Verification items for the finished model (mm, model axes). A direction names the side the tool comes from. Coordinates: 2 decimals unless noted, no trailing zeros. Order: outer loops, then holes, each group sorted by start corner. A loop starts at its lowest first (then second) coordinate and runs counter-clockwise, first axis right, second up. Notation, with made-up numbers: M 57,-6.5 L 65,-6.5 A12 ccw 65,-2.5 Z; hole C -34.75,56 d1. An arc over 180 degrees is marked long. Return JSON: item names as keys, results as strings. Group by question number.
1. Material ranges on line 1 along Z through (x, y) = (-12.75, 1.4); line 2 along X through (y, z) = (0.6, -71.3); line 3 along Z through (x, y) = (-12.75, 1.6), recorded low to high.
2. Gauge pin test, flat ends, axial feed: pin 1 (1.4 mm diameter, centred on x = 8, y = 1.5, fed in from -Z); pin 2 (1.4 mm diameter, centred on y = 1.5, z = -73, fed in from -X). Record the tip position at first contact, or that the pin passes through.
3. Set-up check for faces 3 (the flat face through (-12.8, 1.5, -69.6)), 4 (the flat face through (-1, 0, -1)): record each of +Z, -Z, +X, -X, +Y, -Y from which the full face is reachable in a straight line by a thin tool's end or side.
4. Section check A-A, the plane y = 0.5. Record the cut outline in (x, z).
5. Mould release check, pull along X, two halves, no side actions. Record for faces 1 (the flat face through (-1, 2.8, -1)), 2 (the cylindrical face through (-10.904, 2.159, -67.751)): +X half, -X half, draft (parallel to the pull), parting line (faces both ways), or undercut.
```python
from build123d import *

# Parameters (mm, degrees)
SKETCH1_R           = 1.55
BOSS_EXTRUDE1_DEPTH = 2.8
CUT_EXTRUDE1_REACH  = 4.8
SKETCH2_R           = 1.55
SKETCH3_R           = 4
CUT_EXTRUDE2_DEPTH  = 1.3
CUT_EXTRUDE3_REACH  = 4.8


with BuildPart() as part:
    # Sketch1 → Boss-Extrude1 (new body)
    with BuildSketch(Plane(origin=(0, 0, 0), x_dir=(1, 0, 0), z_dir=(0, 1, 0))):
        Polygon((-72.25, 52), (-72.25, -84), (72.25, -84), (72.25, 84), (-57.25, 84), (-57.25, 52), align=None)
        with Locations((-9.79163056, -53.949747468)):
            Circle(SKETCH1_R, mode=Mode.SUBTRACT)
        with Locations((9.300252532, -73.04163056)):
            Circle(SKETCH1_R, mode=Mode.SUBTRACT)
        with Locations((38.29163056, -44.050252532)):
            Circle(SKETCH1_R, mode=Mode.SUBTRACT)
        with Locations((19.199747468, -24.95836944)):
            Circle(SKETCH1_R, mode=Mode.SUBTRACT)
    extrude(amount=BOSS_EXTRUDE1_DEPTH)

    # Sketch2 → Cut-Extrude1 (cut, up to next)
    with BuildSketch(Plane(origin=(0, 2.8, 0), x_dir=(1, 0, 0), z_dir=(0, 1, 0)), mode=Mode.PRIVATE) as cut_extrude1_sk1:
        with Locations((-12.75, 71.3)):
            Circle(SKETCH2_R)
    cut_extrude1_tool1 = extrude(cut_extrude1_sk1.sketch, amount=-CUT_EXTRUDE1_REACH, mode=Mode.PRIVATE) & part.part
    add(cut_extrude1_tool1.solids().sort_by_distance((-12.75, 2.8, -71.3))[0], mode=Mode.SUBTRACT)
    # Sketch2 → Cut-Extrude1 (cut, up to next)
    with BuildSketch(Plane(origin=(0, 2.8, 0), x_dir=(1, 0, 0), z_dir=(0, 1, 0)), mode=Mode.PRIVATE) as cut_extrude1_sk2:
        with Locations((-12.75, -71.3)):
            Circle(SKETCH2_R)
    cut_extrude1_tool2 = extrude(cut_extrude1_sk2.sketch, amount=-CUT_EXTRUDE1_REACH, mode=Mode.PRIVATE) & part.part
    add(cut_extrude1_tool2.solids().sort_by_distance((-12.75, 2.8, 71.3))[0], mode=Mode.SUBTRACT)

    # Sketch3 → Cut-Extrude2 (cut)
    with BuildSketch(Plane(origin=(0, 2.8, 0), x_dir=(1, 0, 0), z_dir=(0, 1, 0))):
        with Locations((-12.75, 71.3)):
            Circle(SKETCH3_R)
    extrude(amount=-CUT_EXTRUDE2_DEPTH, mode=Mode.SUBTRACT)

    # Sketch4 → Cut-Extrude3 (cut, up to next)
    with BuildSketch(Plane(origin=(0, 2.8, 0), x_dir=(1, 0, 0), z_dir=(0, 1, 0)), mode=Mode.PRIVATE) as cut_extrude3_sk1:
        with BuildLine():
            Line((16.25, 84), (2.25, 84))
            Line((2.25, 84), (2.25, 54))
            ThreePointArc((2.25, 54), (3.128679656, 51.878679656), (5.25, 51))
            Line((5.25, 51), (13.25, 51))
            ThreePointArc((13.25, 51), (15.371320344, 51.878679656), (16.25, 54))
            Line((16.25, 54), (16.25, 84))
        make_face()
    cut_extrude3_tool1 = extrude(cut_extrude3_sk1.sketch, amount=-CUT_EXTRUDE3_REACH, mode=Mode.PRIVATE) & part.part
    add(cut_extrude3_tool1.solids().sort_by_distance((9.25, 2.8, -67.633471))[0], mode=Mode.SUBTRACT)


solid = part.part
```
Answers follow:
{
 "1": {"line 1": "-84 to -72.85, -69.75 to 69.75, 72.85 to 84", "line 2": "-57.25 to -14.3, -11.2 to 2.25, 16.25 to 72.25", "line 3": "-84 to -75.3, -67.3 to 69.75, 72.85 to 84"},
 "2": {"pin 1": "z = -51", "pin 2": "x = -57.25"},
 "3": {"face 3": "+Y", "face 4": "+Z, -Z, +X, -X, -Y"},
 "4": {"outline": "M -72.25,-52 L -57.25,-52 L -57.25,-84 L 2.25,-84 L 2.25,-54 A3 cw 5.25,-51 L 13.25,-51 A3 cw 16.25,-54 L 16.25,-84 L 72.25,-84 L 72.25,84 L -72.25,84 Z; hole C -12.75,-71.3 d3.1; hole C -12.75,71.3 d3.1; hole C -9.79,53.95 d3.1; hole C 9.3,73.04 d3.1; hole C 19.2,24.96 d3.1; hole C 38.29,44.05 d3.1"},
 "5": {"face 1": "draft", "face 2": "undercut"}
}
